Geometry: see drawing. Coordinates: mm, zero at the bounding-box minimum. Give positions to 0.01 mm unless a question says otherwise; leave off trailing zeros. Write each loop counter-clockwise with the first axis right and the second up, starting at its lowest first coordinate (ties: lowest second). Pieces come first, ordered by that corner, then holes. Notation, with made-up numbers: M 9,38 L 27,38 A3 cw 27,43 Z; hole C 55,-13 d5. An arc over 180 degrees is marked long. Use a Markdown table: item, result. Add a question column.
(1) Cut plane C-C (x = 66.5). Output: boundary loops of the cut face in (y, z).
(2) Cut plane B-B (y = 1.8). State how many separate pieces and enclosed holes the cut face has, plus the area to 3 significant figures.
(3) Cut plane A-A (z = 7). Output: boundary loops of the cut face in (x, y).
(4) Pin query (flat end, axial travel): pin 1 Ø2.5 at (x, z) = (29.3, 40) entering from -Y; pin 2 Ø1.5 at (x, y) = (63, 2) entering from -Z; pin 3 Ø1.1 at (x, y) = (75, 0.5) entering from -Z (1 decimal); pin 4 Ø1.5 at (y, z) = (0.5, 40.5) entering from +X. Return the tip coordinate at first contact, or that it passes through.
(5) Cut plane D-D (z = 40). Output: boundary loops of the cut face in (x, y).
(6) Material intervals for L1, parallel to Z at x = 50.7, y = 0.8; L2, parallel to Z at x = 29, y = 2.05; L3, parallel to Z at x = 38, y = 0.6, sorted ascending.
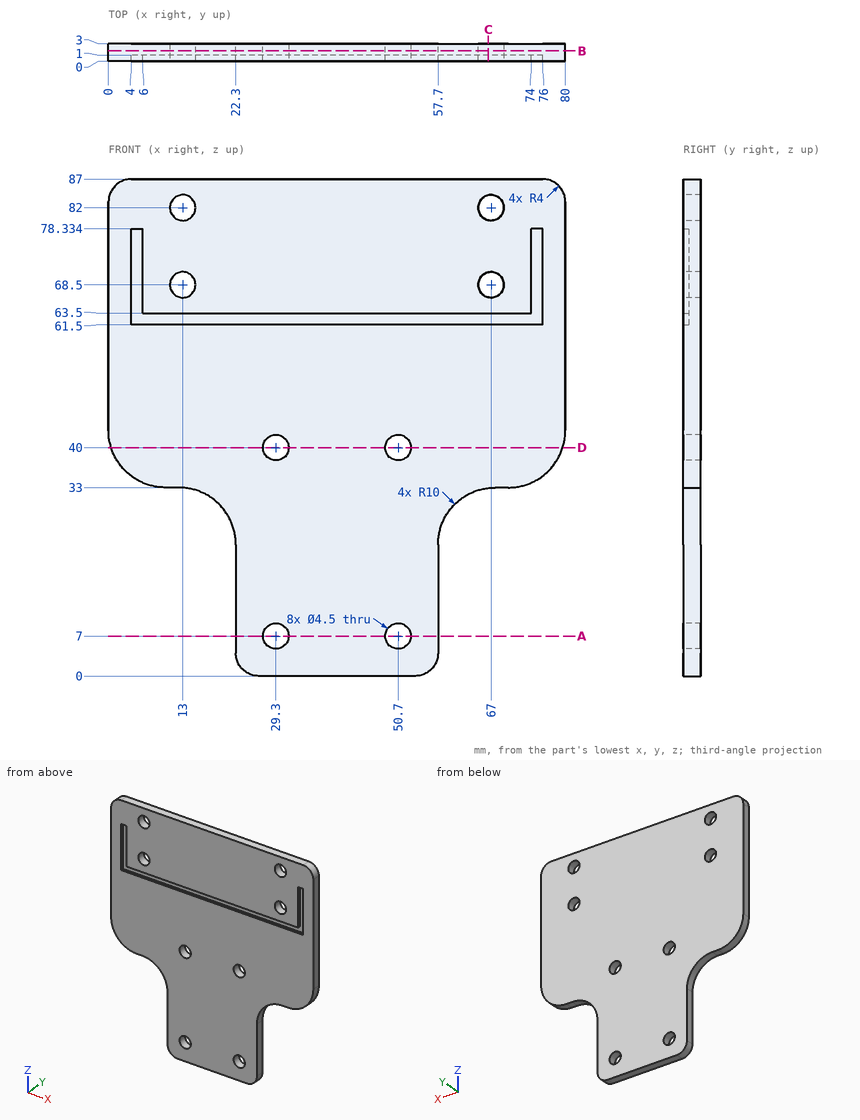
Answer list:
| question | item | result |
|---|---|---|
| 1 | outline | M 0,32.93 L 3,32.93 L 3,66.31 L 0,66.31 L 0,63.5 L 1,63.5 L 1,61.5 L 0,61.5 Z; M 0,70.69 L 3,70.69 L 3,79.81 L 0,79.81 Z; M 0,84.19 L 3,84.19 L 3,87 L 0,87 Z |
| 2 | separate pieces | 1 |
| 2 | enclosed holes | 8 |
| 2 | area | 5,350 mm² |
| 3 | outline | M 22.3,0 L 27.05,0 L 27.05,3 L 22.3,3 Z; M 31.55,0 L 48.45,0 L 48.45,3 L 31.55,3 Z; M 52.95,0 L 57.7,0 L 57.7,3 L 52.95,3 Z |
| 4 | pin 1 | through |
| 4 | pin 2 | z = 31.38 |
| 4 | pin 3 | z = 34 |
| 4 | pin 4 | x = 79.85 |
| 5 | outline | M 0.46,0 L 27.05,0 L 27.05,3 L 0.46,3 Z; M 31.55,0 L 48.45,0 L 48.45,3 L 31.55,3 Z; M 52.95,0 L 79.54,0 L 79.54,3 L 52.95,3 Z |
| 6 | L1 | 0 to 4.75, 9.25 to 37.75, 42.25 to 61.5, 63.5 to 87 |
| 6 | L2 | 0 to 4.77, 9.23 to 37.77, 42.23 to 87 |
| 6 | L3 | 0 to 61.5, 63.5 to 87 |
